Source: three-view drawing plus pictorial views. Frame: mm from the lowest corner of the part. A direction names the side the tool comes from. Coordinates: 2 decimals unless noted, no trailing zeros. Loops run counter-clockwise (first coordinate to the right, second up) from the corner with the lowest first, then second, coordinate; pieces in that order, holes last. Notation, with made-up numbers: (64, 43.5) - (110, 43.5) arc R26 cw to (110, 67.5) - close; hole circle Ø11 at (12, 50.25). An arc over 180 degrees is marked (long way). Return JSON: item names as keys, results as strings.
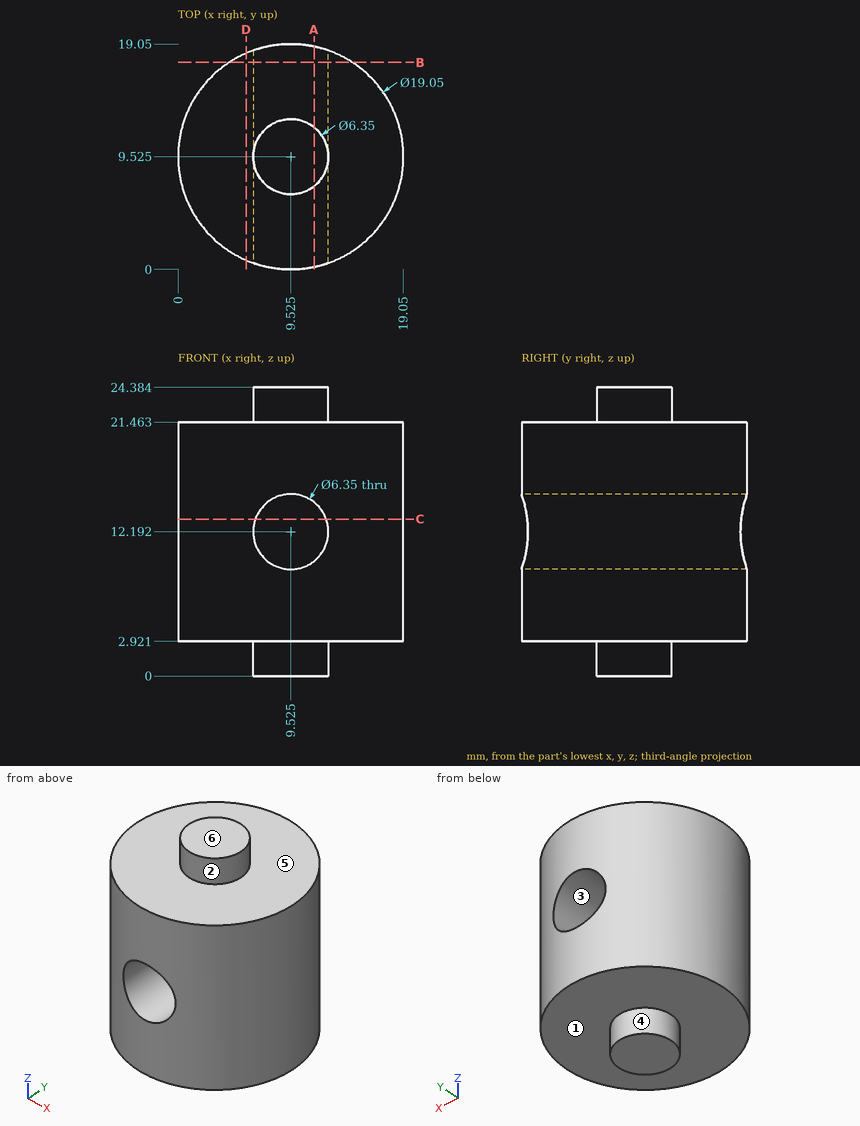
Item 1: Section query A-A, the plane x = 11.5. Return loops of the section in (y, z), and give its area (3 significant figures).
Worked out:
{"outline": "(0.21, 2.92) - (7.04, 2.92) - (7.04, 0) - (12.01, 0) - (12.01, 2.92) - (18.84, 2.92) - (18.84, 9.71) - (0.21, 9.71) - close; (0.21, 14.68) - (18.84, 14.68) - (18.84, 21.46) - (12.01, 21.46) - (12.01, 24.38) - (7.04, 24.38) - (7.04, 21.46) - (0.21, 21.46) - close", "area": "282 mm^2"}
Item 2: Mould query, pull axis Z, two halves, no side actions, for the marked faces 1, 2 and 3. Classes: +Z half, -Z half, draft (parallel to the pull), parting line (faces both ways), or undercut.
Worked out:
{"face 1": "-Z half", "face 2": "draft", "face 3": "undercut"}
Item 3: Section query D-D, the plane x = 5.75. Return loops of the section in (y, z).
Worked out:
{"outline": "(0.78, 2.92) - (18.27, 2.92) - (18.27, 21.46) - (0.78, 21.46) - close"}
Item 4: First-contact query: pin 1 Ø2 at (y, z) = (6.5, 8.5) entering from +X; pin 2 Ø2 at (x, y) = (2, 14) entering from -Z; pin 3 Ø3 at (x, z) = (13, 12) entering from -Y. Flat tips, straight axial feed; report the tip coordinate or a pass-through.
Worked out:
{"pin 1": "x = 18.83", "pin 2": "z = 2.92", "pin 3": "y = 0.42"}
Item 5: Section query B-B, the plane y = 17.5. Return loops of the section in (x, z) (3 decimals), and give its area (3 significant figures).
Worked out:
{"outline": "(4.317, 2.921) - (14.733, 2.921) - (14.733, 21.463) - (4.317, 21.463) - close; hole circle Ø6.35 at (9.525, 12.192)", "area": "161 mm^2"}
Item 6: Ray query, probe 1 along Z at (x, y) = (1, 10.5); probe 2 along Z at (x, y) = (10, 11.75); probe 3 along Z at (x, y) = (10.75, 12). Return the intervals inside material, ascending. Write a range as from..to.
Worked out:
{"probe 1": "2.92..21.46", "probe 2": "0..9.05, 15.33..24.38", "probe 3": "0..9.26, 15.12..24.38"}
Item 7: Reachability of the marked faces 4, 5 and 6 from +Z, -Z, +X, -X, +Y, -Y: full face, straight path, thin tool, end or side. Return the list, or none.
Worked out:
{"face 4": "-Z", "face 5": "+Z", "face 6": "+Z, +X, -X, +Y, -Y"}
Item 8: Section query C-C, the plane z = 13.25. Return loops of the section in (x, y) (3 decimals), and give its area (3 significant figures).
Worked out:
{"outline": "(6.531, 0.483) - (6.531, 18.567) arc R9.525 ccw to start; (12.519, 0.483) arc R9.525 ccw to (12.519, 18.567) - close", "area": "173 mm^2"}
